```python
from build123d import *

# Parameters (mm, degrees)
F0_R      = 6.5
F1_DEPTH  = 4
F2_R      = 4.5
F3_DEPTH  = 1
F4_R      = 4.5
F5_DEPTH  = 1
F6_R      = 1.5
F7_DEPTH  = 1
F8_R      = 1.5
F9_DEPTH  = 1
F10_R     = 1
F11_DEPTH = 25
F13_R     = 8.657699
F13_R_2   = 6
F14_DEPTH = 2


with BuildPart() as f1:
    # F0 (on Top) → F1 (new body)
    with BuildSketch(Plane.XY):
        Circle(F0_R)
    extrude(amount=F1_DEPTH)

    # F2 (on face) → F3 (cut)
    with BuildSketch(Plane(origin=(0, 0, 0), x_dir=(1, 0, 0), z_dir=(0, 0, -1))):
        Circle(F2_R)
    extrude(amount=-F3_DEPTH, mode=Mode.SUBTRACT)

    # F4 (on face) → F5 (cut)
    with BuildSketch(Plane.XY.offset(4)):
        Circle(F4_R)
    extrude(amount=-F5_DEPTH, mode=Mode.SUBTRACT)

    # F6 (on face) → F7 (join)
    with BuildSketch(Plane(origin=(0, 0, 1), x_dir=(1, 0, 0), z_dir=(0, 0, -1))):
        Circle(F6_R)
    extrude(amount=F7_DEPTH)

    # F8 (on face) → F9 (join)
    with BuildSketch(Plane.XY.offset(3)):
        Circle(F8_R)
    extrude(amount=F9_DEPTH)

    # F10 (on face) → F11 (cut)
    with BuildSketch(Plane.XY.offset(4)):
        Circle(F10_R)
    extrude(amount=-F11_DEPTH, mode=Mode.SUBTRACT)

    # F13 (on offset) → F14 (cut)
    with BuildSketch(Plane.XY.offset(1)):
        Circle(F13_R)
        Circle(F13_R_2, mode=Mode.SUBTRACT)
    extrude(amount=F14_DEPTH, mode=Mode.SUBTRACT)


solid = f1.part
```
Geometry: final body of the model. Coordinates: model frame, mm. A direction names the side the tool comes from. Round coordinates to 2 decimals unless told otherwise and drop trailing zeros. Write each loop counter-clockwise with the first axis right and the second up, starting at its lowest first coordinate (ties: lowest second). Pieces come first, ordered by that corner, then holes. Notation, with made-up numbers: M 45,5 L 96,5 A31 ccw 96,41 Z; hole C 19.5,75 d1. An arc over 180 degrees is marked long. Answer in a Markdown table with one row per item. Add a question column.
(1) Reachability of faces 1 (the face through (0, -2, 3)), 2 (the face through (2, -6, 3)), 3 (the face through (-1.5, -0.07, 0.51)) from +Z, -Z, +X, -X, +Y, -Y: full face, straight path, thin tool, end or side. Return the list, or none.
(2) Contact query for flat-ended pins moving along their axis: pin 1 (1.5 mm diameter, centred on y = 1.5, z = 2.5, fed in from +X); pin 2 (4 mm diameter, centred on x = -2.5, y = 1.5, fed in from -Z). Output: stop coordinate, or through.
(3) Ray query, L1, parallel to Y at x = 0, z = 3.7; L2, parallel to Y at x = 0, z = 2.9; L3, parallel to Z at x = 4.25, y = -4.5. Return the intervals inside material, ascending.
(4) Cut plane D-D, the plane y = -2.5. Return the cut outline in (x, z), then the cut area to 3 significant figures.
(5) Draft query along Y for faces 4 (the face through (-6, 0, 2)), 5 (the face through (-1.5, 0.07, 3.49)), 6 (the face through (-4.42, 1.54, 0)). Return one class per face: pulls with the +Y half, pulls with the -Y half, needs draft (parallel to the pull), parting line crosses it, or undercut.
(6) Cut plane C-C, the plane z = 3.8. Return the cut outline in (x, y), then the cut area to 3 significant figures.
Established:
| question | item | result |
|---|---|---|
| 1 | face 1 | +Z |
| 1 | face 2 | none |
| 1 | face 3 | -Z |
| 2 | pin 1 | x = 6.43 |
| 2 | pin 2 | z = 0 |
| 3 | L1 | -6.5 to -4.5, -1.5 to -1, 1 to 1.5, 4.5 to 6.5 |
| 3 | L2 | -6 to -1, 1 to 6 |
| 3 | L3 | 0 to 1, 3 to 4 |
| 4 | outline | M -6,0 L -3.74,0 L -3.74,1 L 3.74,1 L 3.74,0 L 6,0 L 6,1 L 5.45,1 L 5.45,3 L 6,3 L 6,4 L 3.74,4 L 3.74,3 L -3.74,3 L -3.74,4 L -6,4 L -6,3 L -5.45,3 L -5.45,1 L -6,1 Z |
| 4 | area | 30.9 mm² |
| 5 | face 4 | parting line crosses it |
| 5 | face 5 | undercut |
| 5 | face 6 | needs draft |
| 6 | outline | C 0,0 d13; C 0,0 d3; hole C 0,0 d9; hole C 0,0 d2 |
| 6 | area | 73.0 mm² |
